from build123d import *

# Parameters (mm, degrees)
F1_W     = 90
F1_H     = 53
F1_W_2   = 35
F1_H_2   = 15
F2_DEPTH = 1.5
F3_W     = 90
F3_H     = 53
F3_W_2   = 87
F3_H_2   = 50
F4_DEPTH = 4.6
F5_W     = 38
F5_H     = 18
F5_W_2   = 35
F5_H_2   = 15
F6_DEPTH = 3
F7_R     = 0.5


with BuildPart() as f2:
    # F1 (on Top) → F2 (new body)
    with BuildSketch(Plane.XY):
        Rectangle(F1_W, F1_H)
        Rectangle(F1_W_2, F1_H_2, mode=Mode.SUBTRACT)
    extrude(amount=F2_DEPTH)

    # F3 (on face) → F4 (join)
    with BuildSketch(Plane.XY.offset(1.5)):
        Rectangle(F3_W, F3_H)
        Rectangle(F3_W_2, F3_H_2, mode=Mode.SUBTRACT)
    extrude(amount=F4_DEPTH)

    # F5 (on face) → F6 (join)
    with BuildSketch(Plane.XY.offset(1.5)):
        Polygon((-38.5, 25), (-43.5, 25), (-43.5, 20), align=None)
        Polygon((43.5, 20), (43.5, 25), (38.5, 25), align=None)
        Polygon((-43.5, -20), (-43.5, -25), (-38.5, -25), align=None)
        Polygon((38.5, -25), (43.5, -25), (43.5, -20), align=None)
        Rectangle(F5_W, F5_H)
        Rectangle(F5_W_2, F5_H_2, mode=Mode.SUBTRACT)
    extrude(amount=F6_DEPTH)

    # F7
    f7_edges = [f2.edges().sort_by_distance(p)[0] for p in [
        (-45, -26.5, 3.05),
        (45, -26.5, 3.05),
        (45, 26.5, 3.05),
        (-45, 26.5, 3.05),
        (0, 26.5, 6.1),
        (-45, 0, 6.1),
        (45, 0, 6.1),
        (0, -26.5, 6.1),
        (-43.5, 0, 6.1),
        (0, 25, 6.1),
        (43.5, 0, 6.1),
        (0, -25, 6.1),
        (0, -9, 4.5),
        (19, 0, 4.5),
        (0, 7.5, 4.5),
        (0, 9, 4.5),
        (17.5, 0, 4.5),
        (-17.5, 0, 4.5),
        (-19, 0, 4.5),
        (0, 7.5, 0),
        (-17.5, 0, 0),
        (0, -7.5, 0),
        (17.5, 0, 0),
        (-19, -9, 3),
        (-19, 9, 3),
        (-19, 0, 1.5),
        (0, -7.5, 4.5),
        (19, 0, 1.5),
        (19, 9, 3),
        (19, -9, 3),
        (-43.5, 0, 1.5),
        (-41, -22.5, 1.5),
        (-41, 22.5, 1.5),
        (0, 25, 1.5),
        (41, 22.5, 1.5),
        (43.5, 0, 1.5),
        (41, -22.5, 1.5),
        (0, -25, 1.5),
        (0, 9, 1.5),
        (0, -9, 1.5),
    ]]
    fillet(f7_edges, radius=F7_R)


solid = f2.part
Work out the finished part from the listing and answer in its coordinate system (mm). A direction names the side the tool comes from. Round coordinates to 2 decimals unless told otherwise and drop trailing zeros. Write each loop counter-clockwise with the first axis right and the second up, starting at its lowest first coordinate (ties: lowest second). Pieces come first, ordered by that corner, then holes. Notation, with made-up numbers: M 43,61 L 88,61 A4 ccw 88,65 Z; hole C 79,74.25 d11. An arc over 180 degrees is marked long. Use a Markdown table: item, result.
1) Determine the mould class of faces 1 (the face through (-45, 0, 3)), 2 (the face through (-17.5, 0, 2)) for opening direction X: pulls with the +X half, pulls with the -X half, needs draft (parallel to the pull), parting line crosses it, or undercut.
Taken from the geometry:
| item | result |
|---|---|
| face 1 | pulls with the -X half |
| face 2 | undercut |
2) The part is cut by section C-C on y = 18. Give the vertices of the cut face in (x, z), plus the area to 3 significant figures.
Taken from the geometry:
| item | result |
|---|---|
| outline | M -45,0 L 45,0 L 45,5.6 A0.5 ccw 44.5,6.1 L 44,6.1 A0.5 ccw 43.5,5.6 L 43.5,2 A0.5 cw 43,1.5 L -43,1.5 A0.5 cw -43.5,2 L -43.5,5.6 A0.5 ccw -44,6.1 L -44.5,6.1 A0.5 ccw -45,5.6 Z |
| area | 149 mm2 |
3) The part is cut by section D-D on x = 36. Give the vertices of the cut face in (y, z), plus the area to 3 significant figures.
Taken from the geometry:
| item | result |
|---|---|
| outline | M -26.5,0 L 26.5,0 L 26.5,5.6 A0.5 ccw 26,6.1 L 25.5,6.1 A0.5 ccw 25,5.6 L 25,2 A0.5 cw 24.5,1.5 L -24.5,1.5 A0.5 cw -25,2 L -25,5.6 A0.5 ccw -25.5,6.1 L -26,6.1 A0.5 ccw -26.5,5.6 Z |
| area | 93.2 mm2 |
4) Consider line 1 (Y direction, x = -18, z = 2.25); line 2 (Y direction, x = -15.5, z = 3); line 3 (X direction, y = -17.5, z = 3.5). Determine where each line is inside the solid, lowest interval first. Write a range as [from, to].
Taken from the geometry:
| item | result |
|---|---|
| line 1 | y = [-26.5, -25], [-9, 9], [25, 26.5] |
| line 2 | y = [-26.5, -25], [-9, -7.5], [7.5, 9], [25, 26.5] |
| line 3 | x = [-45, -43.5], [43.5, 45] |
5) Flat-ended cylindrical pins translate along their axes: pin 1 (5.5 mm diameter, centred on x = 40.5, y = 22, fed in from +Z); pin 2 (5 mm diameter, centred on x = -14.5, y = -14, fed in from +Z). Find the tip coordinate at first contact, or state that the pin passes through.
Taken from the geometry:
| item | result |
|---|---|
| pin 1 | stops at z = 4.5 |
| pin 2 | stops at z = 1.5 |
6) Which of the six approach directions +Z, -Z, +X, -X, +Y, -Y give full straight-line access (tool end or side, diameter ignored) to faces 3 (the face through (-40.864, 22.434, 1.65)), 4 (the face through (0, 7.5, 2))?
Taken from the geometry:
| item | result |
|---|---|
| face 3 | +Z |
| face 4 | +Z, -Z |
